Geometry check sheet. Reference: the model listing, model coordinates, mm. A direction names the side the tool comes from. Round coordinates to 2 decimals unless told otherwise and drop trailing zeros. Write each loop counter-clockwise with the first axis right and the second up, starting at its lowest first coordinate (ties: lowest second). Pieces come first, ordered by that corner, then holes. Notation, with made-up numbers: M 20.5,70 L 69.5,70 A11 cw 69.5,75 Z; hole C 7,28.25 d6. An arc over 180 degrees is marked long. Use a Markdown table: item, result.
```python
from build123d import *

# Parameters (mm, degrees)
F0_R             = 6.35
F1_DEPTH         = 12.7
F4_R             = 7.62
F6_DEPTH         = 5.08
F6_COPIES_COUNT  = 2
F6_COPIES_PITCH  = 14.929745
F6_COPIES1_COUNT = 2
F6_COPIES1_PITCH = 14.929745
F6_COPIES2_COUNT = 2
F6_COPIES2_PITCH = 24.156836
F6_COPIES3_COUNT = 2
F6_COPIES3_PITCH = 24.156836


# Not quite as in the source:
# - a pattern or mirror of a feature is missing from the dataset's text; its kind, count and spacing are read off the source's solid


with BuildPart() as f1:
    # F0 (on Top) → F1 (new body)
    with BuildSketch(Plane.XY):
        with BuildLine():
            Line((0, 31.75), (0, 6.35))
            Line((0, 6.35), (12.7, 6.35))
            ThreePointArc((12.7, 6.35), (17.1901280605, 4.4901280605), (19.05, 0))
            Line((19.05, 0), (114.3, 0))
            Line((114.3, 0), (114.3, 31.75))
            ThreePointArc((114.3, 31.75), (101.6, 44.45), (88.9, 31.75))
            Line((88.9, 31.75), (88.9, 19.05))
            Line((88.9, 19.05), (25.4, 19.05))
            Line((25.4, 19.05), (25.4, 31.75))
            ThreePointArc((25.4, 31.75), (12.7, 44.45), (0, 31.75))
        make_face()
        with Locations((12.7, 31.75)):
            Circle(F0_R, mode=Mode.SUBTRACT)
        with Locations((101.6, 31.75)):
            Circle(F0_R, mode=Mode.SUBTRACT)
    extrude(amount=F1_DEPTH)

    # F2: F1 across plane


with BuildPart() as f1_1:
    add(f1.part)
    add(f1.part.mirror(Plane.XZ))

    # F4 (on face) → F5 (join, up to the next surface of F1)
    with BuildSketch(Plane(origin=(63.5, 0, 63.5), x_dir=(0, 1, 0), z_dir=(0.7071067812, 0, 0.7071067812))):
        with BuildLine():
            Line((-19.05, -36.9170489686), (-19.05, -71.8420489686))
            Line((-19.05, -71.8420489686), (19.05, -71.8420489686))
            Line((19.05, -71.8420489686), (19.05, -36.9170489686))
            ThreePointArc((19.05, -36.9170489686), (0, -17.8670489686), (-19.05, -36.9170489686))
        make_face()
        with BuildLine():
            ThreePointArc((-2.5272680903, -24.4710489686), (-0.1271594487, -21.6802339429), (2.54, -24.2170489686))
            ThreePointArc((2.54, -24.2170489686), (2.5368150257, -24.3442084172), (2.5272680903, -24.4710489686))
            ThreePointArc((2.5272680903, -24.4710489686), (9.8332676346, -28.8798325582), (12.7, -36.9170489686))
            ThreePointArc((12.7, -36.9170489686), (-8.0372164104, -46.7503166031), (-2.5272680903, -24.4710489686))
        make_face(mode=Mode.SUBTRACT)
        with BuildLine():
            ThreePointArc((2.5272680903, -24.4710489686), (0, -26.7570489686), (-2.5272680903, -24.4710489686))
            ThreePointArc((-2.5272680903, -24.4710489686), (-8.0372164104, -46.7503166031), (12.7, -36.9170489686))
            ThreePointArc((12.7, -36.9170489686), (9.8332676346, -28.8798325582), (2.5272680903, -24.4710489686))
        make_face()
        with Locations((0, -36.9170489686)):
            Circle(F4_R, mode=Mode.SUBTRACT)
        with BuildLine():
            ThreePointArc((2.5272680903, -24.4710489686), (2.5368150257, -24.3442084172), (2.54, -24.2170489686))
            ThreePointArc((2.54, -24.2170489686), (-0.1271594487, -21.6802339429), (-2.5272680903, -24.4710489686))
            ThreePointArc((-2.5272680903, -24.4710489686), (0, -24.2170489686), (2.5272680903, -24.4710489686))
        make_face()
        with BuildLine():
            ThreePointArc((2.5272680903, -24.4710489686), (0, -24.2170489686), (-2.5272680903, -24.4710489686))
            ThreePointArc((-2.5272680903, -24.4710489686), (0, -26.7570489686), (2.5272680903, -24.4710489686))
        make_face()
    extrude(until=Until.NEXT, dir=(-0.7071067812, 0, -0.7071067812))

    # F4 (on face) → F6 (cut)
    with BuildSketch(Plane(origin=(63.5, 0, 63.5), x_dir=(0, 1, 0), z_dir=(0.7071067812, 0, 0.7071067812))):
        with BuildLine():
            ThreePointArc((2.5272680903, -24.4710489686), (2.5368150257, -24.3442084172), (2.54, -24.2170489686))
            ThreePointArc((2.54, -24.2170489686), (-0.1271594487, -21.6802339429), (-2.5272680903, -24.4710489686))
            ThreePointArc((-2.5272680903, -24.4710489686), (0, -24.2170489686), (2.5272680903, -24.4710489686))
        make_face()
        with BuildLine():
            ThreePointArc((2.5272680903, -24.4710489686), (0, -24.2170489686), (-2.5272680903, -24.4710489686))
            ThreePointArc((-2.5272680903, -24.4710489686), (0, -26.7570489686), (2.5272680903, -24.4710489686))
        make_face()
    f6 = extrude(amount=-F6_DEPTH, mode=Mode.SUBTRACT)

    # F6_copies: F6 ×2
    with Locations(*[Vector(0.4156269378, 0.8090169944, -0.4156269378) * (i * F6_COPIES_PITCH) for i in range(1, F6_COPIES_COUNT)]):
        add(f6, mode=Mode.SUBTRACT)

    # F6_copies1: F6 ×2
    with Locations(*[Vector(0.4156269378, -0.8090169944, -0.4156269378) * (i * F6_COPIES1_PITCH) for i in range(1, F6_COPIES1_COUNT)]):
        add(f6, mode=Mode.SUBTRACT)

    # F6_copies2: F6 ×2
    with Locations(*[Vector(0.672498512, -0.3090169944, -0.672498512) * (i * F6_COPIES2_PITCH) for i in range(1, F6_COPIES2_COUNT)]):
        add(f6, mode=Mode.SUBTRACT)

    # F6_copies3: F6 ×2
    with Locations(*[Vector(0.672498512, 0.3090169944, -0.672498512) * (i * F6_COPIES3_PITCH) for i in range(1, F6_COPIES3_COUNT)]):
        add(f6, mode=Mode.SUBTRACT)


solid = f1_1.part
```
Item 1: Cross-section at B-B, the plane z = 8.5. Record the cut outline in (x, y).
Outcome:
| item | result |
|---|---|
| outline | M 0,-31.75 A12.7 ccw 25.4,-31.75 L 25.4,-19.05 L 88.9,-19.05 L 88.9,-31.75 A12.7 ccw 114.3,-31.75 L 114.3,31.75 A12.7 ccw 88.9,31.75 L 88.9,19.05 L 25.4,19.05 L 25.4,31.75 A12.7 ccw 0,31.75 L 0,6.35 L 12.7,6.35 A6.35 cw 12.7,-6.35 L 0,-6.35 Z; hole C 12.7,-31.75 d12.7; hole C 12.7,31.75 d12.7; hole C 101.6,-31.75 d12.7; hole C 101.6,31.75 d12.7 |
Item 2: Access from +Z, -Z, +X, -X, +Y, -Y to the whole of each face (thin tool, end or side, straight path). Record for faces 1 (the face through (101, -23, 12.7)), 2 (the face through (25.4, 25, 6)), 3 (the face through (83.212, -12.114, 36.604)), 4 (the face through (6, 6.35, 6)).
Outcome:
| item | result |
|---|---|
| face 1 | +Z, +X, -X, -Y |
| face 2 | +Z, -Z, +Y |
| face 3 | none |
| face 4 | +Z, -Z, -X |
Item 3: Mould release check, pull along Z, two halves, no side actions. Record for faces 5 (the face through (101.879, 44.447, 6.261)), 6 (the face through (65, 0, 12.7)), 7 (the face through (99, 0, 28)), 8 (the face through (72.773, -0.992, 31.249)): +Z half, -Z half, draft (parallel to the pull), parting line (faces both ways), or undercut.
Outcome:
| item | result |
|---|---|
| face 5 | draft |
| face 6 | undercut |
| face 7 | +Z half |
| face 8 | undercut |
Item 4: Go/stop test with flat-tipped pins: pin 1 (1.5 mm diameter, centred on x = 57, z = 25.5, fed in from +Y); pin 2 (6 mm diameter, centred on x = 63, z = 39, fed in from -Y); pin 3 (5 mm diameter, centred on y = -7.5, z = 19.5, fed in from +X). Record where each tip stops, or that it passes through.
Outcome:
| item | result |
|---|---|
| pin 1 | stops at y = 13.03 |
| pin 2 | stops at y = -8.7 |
| pin 3 | stops at x = 110 |
Item 5: Material ranges on line 1 along X through (y, z) = (-31.75, 3); line 2 along Y through (x, z) = (12.7, 8); line 3 along Y through (x, z) = (101.6, 9.5), recorded low to high. Write a range as from..to.
Outcome:
| item | result |
|---|---|
| line 1 | x = 0..6.35, 19.05..25.4, 88.9..95.25, 107.95..114.3 |
| line 2 | y = -44.45..-38.1, -25.4..-6.35, 6.35..25.4, 38.1..44.45 |
| line 3 | y = -44.45..-38.1, -25.4..25.4, 38.1..44.45 |
Item 6: Cross-section at C-C, the plane y = -30. Record the cut outline in (x, z), and give its area (3 significant figures).
Outcome:
| item | result |
|---|---|
| outline | M 0,0 L 6.6,0 L 6.6,12.7 L 0,12.7 Z; M 18.8,0 L 25.4,0 L 25.4,12.7 L 18.8,12.7 Z; M 88.9,0 L 95.5,0 L 95.5,12.7 L 88.9,12.7 Z; M 107.7,0 L 114.3,0 L 114.3,12.7 L 107.7,12.7 Z |
| area | 335 mm2 |
Item 7: Cross-section at D-D, the plane y = 16. Record the cut outline in (x, z), and give its area (3 significant figures).
Outcome:
| item | result |
|---|---|
| outline | M 0,0 L 114.3,0 L 114.3,12.7 L 82.29,44.71 L 50.29,12.7 L 0,12.7 Z |
| area | 2,480 mm2 |
Item 8: Cross-section at A-A, the plane x = 101.6. Record the cut outline in (y, z).
Outcome:
| item | result |
|---|---|
| outline | M -44.45,0 L -38.1,0 L -38.1,12.7 L -44.45,12.7 Z; M -25.4,0 L 25.4,0 L 25.4,12.7 L 19.05,12.7 L 19.05,25.4 L -19.05,25.4 L -19.05,12.7 L -25.4,12.7 Z; M 38.1,0 L 44.45,0 L 44.45,12.7 L 38.1,12.7 Z |
